```python
from build123d import *

# Parameters (mm, degrees)
BOSS_EXTRUDE1_DEPTH = 1.5
FILLET1_R           = 1.5875
SKETCH2_W           = 3
SKETCH2_H           = 6.35
BOSS_EXTRUDE2_DEPTH = 3
FILLET2_R           = 0.79375
FILLET3_R           = 1.27


with BuildPart() as part:
    # Sketch1 → Boss-Extrude1 (new, symmetric)
    with BuildSketch(Plane(origin=(0, 0, 0), x_dir=(1, 0, 0), z_dir=(0, 1, 0))):
        Polygon((25.4, 19.05), (9.525, 19.05), (9.525, -19.05), (25.4, -19.05), (25.4, -31.75), (-25.4, -31.75), (-25.4, -19.05), (-9.525, -19.05), (-9.525, 19.05), (-25.4, 19.05), (-25.4, 31.75), (-9.525, 31.75), (-9.525, 30.48), (9.525, 30.48), (9.525, 31.75), (25.4, 31.75), align=None)
    extrude(amount=BOSS_EXTRUDE1_DEPTH, both=True)

    # Fillet1
    fillet1_edges = [part.edges().sort_by_distance(p)[0] for p in [
        (25.4, 0, -31.75),
        (25.4, 0, -19.05),
        (9.525, 0, -19.05),
        (9.525, 0, 19.05),
        (25.4, 0, 19.05),
        (25.4, 0, 31.75),
        (-25.4, 0, 31.75),
        (-25.4, 0, 19.05),
        (-9.525, 0, 19.05),
        (-9.525, 0, -19.05),
        (-25.4, 0, -19.05),
        (-25.4, 0, -31.75),
    ]]
    fillet(fillet1_edges, radius=FILLET1_R)

    # Sketch2 → Boss-Extrude2 (add)
    with BuildSketch(Plane(origin=(0, 1.5, 0), x_dir=(1, 0, 0), z_dir=(0, 1, 0))):
        with Locations((-26.9, 25.4)):
            Rectangle(SKETCH2_W, SKETCH2_H)
        with Locations((26.9, 25.4)):
            Rectangle(SKETCH2_W, SKETCH2_H)
        with Locations((26.9, -25.4)):
            Rectangle(SKETCH2_W, SKETCH2_H)
        with Locations((-26.9, -25.4)):
            Rectangle(SKETCH2_W, SKETCH2_H)
    extrude(amount=-BOSS_EXTRUDE2_DEPTH)

    # Fillet2
    fillet2_edges = [part.edges().sort_by_distance(p)[0] for p in [
        (-28.4, 0, 28.575),
        (-28.4, 0, 22.225),
        (28.4, 0, 22.225),
        (28.4, 0, 28.575),
        (28.4, 0, -28.575),
        (28.4, 0, -22.225),
        (-28.4, 0, -22.225),
        (-28.4, 0, -28.575),
    ]]
    fillet(fillet2_edges, radius=FILLET2_R)

    # Fillet3
    fillet3_edges = [part.edges().sort_by_distance(p)[0] for p in [
        (9.525, 0, -31.75),
        (-9.525, 0, -31.75),
    ]]
    fillet(fillet3_edges, radius=FILLET3_R - 0.0001)  # a hair under: the kernel refuses the full size


solid = part.part
```
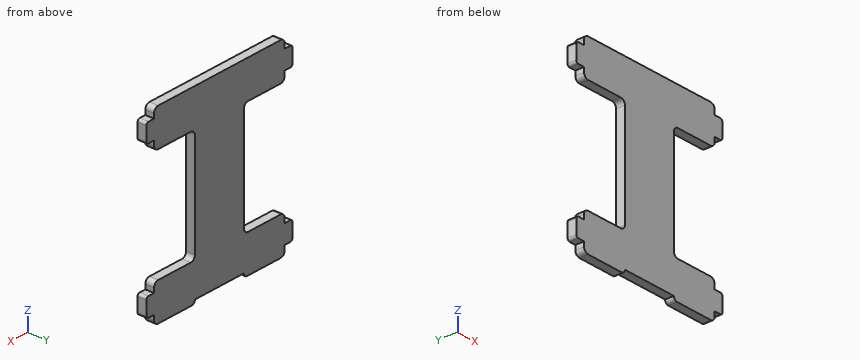
Here's how the part is built. I have some questions about the finished solid (model axes, mm). Coordinates: 2 decimals unless noted, no trailing zeros. Loops run counter-clockwise (first coordinate to the right, second up) from the corner with the lowest first, then second, coordinate; pieces in that order, holes last. Notation, with made-up numbers: M -29.75,18.5 L -10.75,18.5 A31 cw -10.75,52.5 Z; hole C 78,56 d9. An arc over 180 degrees is marked long. One line per item, written item: value.
1. Imagine slicing it at A-A (x = 15). List the corners of the cut face in (y, z) for me, and give its area (3 significant figures).
Geometry says:
outline: M -1.5,-31.75 L 1.5,-31.75 L 1.5,-19.05 L -1.5,-19.05 Z; M -1.5,19.05 L 1.5,19.05 L 1.5,31.75 L -1.5,31.75 Z
area: 76.2 mm2
2. Imagine slicing it at B-B (z = -7). List the corners of the cut face in (x, y) for me (3 decimals).
Geometry says:
outline: M -9.525,-1.5 L 9.525,-1.5 L 9.525,1.5 L -9.525,1.5 Z
3. Please list where these lines run through material, in increasing order: probe 1 along Z at (x, y) = (14, 0.3); probe 2 along X at (y, z) = (-0.75, 15) (3 decimals); probe 3 along Z at (x, y) = (-9, -0.6).
Geometry says:
probe 1: z = -31.75 to -19.05, 19.05 to 31.75
probe 2: x = -9.525 to 9.525
probe 3: z = -30.48 to 31.75
4. Imagine slicing it at C-C (x = 2.5). List the corners of the cut face in (y, z) for me.
Geometry says:
outline: M -1.5,-30.48 L 1.5,-30.48 L 1.5,31.75 L -1.5,31.75 Z
5. Imagine slicing it at D-D (x = 24.5). List the corners of the cut face in (y, z) for me, and give its area (3 significant figures).
Geometry says:
outline: M -1.5,-31.59 L 1.5,-31.59 L 1.5,-19.21 L -1.5,-19.21 Z; M -1.5,19.21 L 1.5,19.21 L 1.5,31.59 L -1.5,31.59 Z
area: 74.3 mm2
6. Will these pins go through, and if not, where does the flat tip stop? pin 1 Ø1.7 at (y, z) = (-0.5, -21) entering from -X; pin 2 Ø1.7 at (y, z) = (-0.5, 29) entering from -X; pin 3 Ø1.5 at (y, z) = (0.5, 4) entering from +X (3 decimals).
Geometry says:
pin 1: stops at x = -25.4
pin 2: stops at x = -28.31
pin 3: stops at x = 9.525
